Autodesk Inventor part; units mm, degrees
ref_plane "YZ Plane" through (0, 0, 0) normal (1, 0, 0) x (0, 1, 0)
ref_plane "XZ Plane" through (0, 0, 0) normal (0, 1, 0) x (-1, 0, 0)
ref_plane "XY Plane" through (0, 0, 0) normal (0, 0, 1) x (1, 0, 0)
sketch "Sketch1" plane through (0, 0, 0) normal (0, 0, 1) x (1, 0, 0)
  circle A0 centre (0, 15.825) radius 9.125
  line L0 (-12.375, 0) -> (12.375, 0)
  arc A1 (12.375, 15.825) -> (-12.375, 15.825) centre (0, 15.825) ccw
  line L1 (12.375, 0) -> (12.375, 15.825)
  line L2 (-12.375, 0) -> (-12.375, 15.825)
  point P0 (0, 0)
  point P1 (0, 0)
  point P2 (0, 0)
  point P3 (0, 3.45)
  dimension "d28" = 18.25
  dimension "d29" = 24.75
  dimension "d30" = 24.75
  dimension "d31" = 3.45
sketch "Sketch2" plane through (0, 0, 0) normal (0, 1, 0) x (-1, 0, 0)
  line L0 (12.375, 0) -> (-12.375, 0)
  line L1 (-12.375, 0) -> (-12.375, -10)
  line L2 (-12.375, -10) -> (12.375, -10)
  line L3 (12.375, -10) -> (12.375, 0)
  point P0 (0, 0)
  point P1 (-12.375, 0)
  dimension "d5" = 24.75
  dimension "d10" = 10
extrude "Extrusion4" add sketch "Sketch2" along normal blind 2
extrude "Extrusion5" add sketch "Sketch1" against normal blind 2
hole "Hole2" at (-8.875, 2, -6.5) direction (0, -1, 0) diameter 2.25 end through all
pattern_linear "Rectangular Pattern2" count 2 spacing 17.75 along (1, 0, 0) of "Hole2"
fillet "Fillet1" radius 0.5 2 edges at (0, 0, 0) (0, 2, -2)
properties part number "DudukanProximity"
The listing builds one solid part. Answer for the finished solid, in the listing's coordinates (mm). A direction names the side the tool comes from. Give positions to 0.01 mm unless a question says otherwise; leave off trailing zeros. Loops run counter-clockwise (first coordinate to the right, second up) from the corner with the lowest first, then second, coordinate; pieces in that order, holes last. Notation, with made-up numbers: M 50.25,39 L 86.25,39 A30 cw 86.25,69 Z; hole C 44.25,61.5 d5. An arc over 180 degrees is marked long. One line per item, written item: value.
Q1. Flat-ended cylindrical pins translate along their axes: P1, Ø3, axis at x = 8.875, z = -6.5, coming from the +Y side; P2, Ø8, axis at x = 7.5, y = 7, coming from the +Z side; P3, Ø7.5, axis at x = -3, y = 14.5, coming from the -Z side. Find the tip coordinate at first contact, or state that the pin passes through.
Working result:
P1: stops at y = 2
P2: stops at z = 0
P3: passes through
Q2. A cutting plane is placed at B-B on z = -6.5. Determine the outline of the cut face in (x, y) (3 decimals), then the cut area to 3 significant figures.
Working result:
outline: M -12.375,0 L -10,0 L -10,2 L -12.375,2 Z; M -7.75,0 L 7.75,0 L 7.75,2 L -7.75,2 Z; M 10,0 L 12.375,0 L 12.375,2 L 10,2 Z
area: 40.5 mm^2
Q3. A cutting plane is placed at D-D on x = -6.75. Determine the outline of the cut face in (y, z), then the cut area to 3 significant figures.
Working result:
outline: M 0,-10 L 2,-10 L 2,-2.5 A0.5 cw 2.5,-2 L 9.68,-2 L 9.68,0 L 0.5,0 A0.5 ccw 0,-0.5 Z; M 21.97,-2 L 26.2,-2 L 26.2,0 L 21.97,0 Z
area: 43.8 mm^2
Q4. Determine the mould class of faces 1 (the face through (0, 1, -10)), 2 (the face through (0, 2, -6)), 3 (the face through (-7.777, 0.986, -6.744)), 4 (the face through (9.973, 0.986, -6.744)) for opening direction Z: +Z half, -Z half, draft (parallel to the pull), parting line (faces both ways), or undercut.
Working result:
face 1: -Z half
face 2: draft
face 3: undercut
face 4: undercut
Q5. A cutting plane is placed at C-C on y = 20.25. Determine the outline of the cut face in (x, z).
Working result:
outline: M -11.56,-2 L -7.98,-2 L -7.98,0 L -11.56,0 Z; M 7.98,-2 L 11.56,-2 L 11.56,0 L 7.98,0 Z
Q6. For faces 5 (the face through (4.906, 23.519, -0.986)), 6 (the face through (3, 7, -2)), determine the directions among +Z, -Z, +X, -X, +Y, -Y from which every point of the face is accessible in a straight line to the end or side of a thin tool.
Working result:
face 5: +Z, -Z
face 6: -Z, +X, -X, +Y
Q7. A cutting plane is placed at A-A on x = 0. Determine the outline of the cut face in (y, z).
Working result:
outline: M 0,-10 L 2,-10 L 2,-2.5 A0.5 cw 2.5,-2 L 6.7,-2 L 6.7,0 L 0.5,0 A0.5 ccw 0,-0.5 Z; M 24.95,-2 L 28.2,-2 L 28.2,0 L 24.95,0 Z
Q8. Find the intervals of material crossed by line 1 (X direction, y = 1.4, z = -6.5) (3 decimals); line 2 (Y direction, x = 0, z = -0.9); line 3 (Y direction, x = -1, z = -4.5), in increasing order. Write a range as from..to.
Working result:
line 1: x = -12.375..-10, -7.75..7.75, 10..12.375
line 2: y = 0..6.7, 24.95..28.2
line 3: y = 0..2
